from build123d import *

# Parameters (mm, degrees)
SKETCH_1_W          = 390
SKETCH_1_H          = 250
EXTRUDE_1_DEPTH     = 2
SKETCH_2_W          = 130
SKETCH_2_H          = 40
SKETCH_2_W_2        = 125
SKETCH_2_H_2        = 60
CUT_EXTRUDE_1_DEPTH = 5
CUT_EXTRUDE_2_DEPTH = 10
FILLET_1_R          = 5
SKETCH_4_R          = 1.5
SKETCH_4_R_2        = 1.75
CUT_EXTRUDE_3_DEPTH = 232.633330935
SKETCH_5_R          = 1.75
CUT_EXTRUDE_4_DEPTH = 232.633330935


with BuildPart() as part:
    # 스케치1 → 보스-돌출1 (new body)
    with BuildSketch(Plane(origin=(0, 0, 0), x_dir=(1, 0, 0), z_dir=(0, 1, 0))):
        Rectangle(SKETCH_1_W, SKETCH_1_H)
    extrude(amount=EXTRUDE_1_DEPTH)

    # 스케치2 → 컷-돌출1 (cut)
    with BuildSketch(Plane(origin=(0, 2, 0), x_dir=(1, 0, 0), z_dir=(0, 1, 0))):
        with Locations((-85, 105)):
            Rectangle(SKETCH_2_W, SKETCH_2_H)
        with Locations((-85, -105)):
            Rectangle(SKETCH_2_W, SKETCH_2_H)
        with Locations((132.5, 95)):
            Rectangle(SKETCH_2_W_2, SKETCH_2_H_2)
        with Locations((132.5, -95)):
            Rectangle(SKETCH_2_W_2, SKETCH_2_H_2)
    extrude(amount=-CUT_EXTRUDE_1_DEPTH, mode=Mode.SUBTRACT)

    # 스케치3 → 컷-돌출2 (cut)
    with BuildSketch(Plane(origin=(0, 2, 0), x_dir=(1, 0, 0), z_dir=(0, 1, 0))):
        Polygon((-5, 125), (70, 65), (70, 125), align=None)
        Polygon((70, -65), (-5, -125), (70, -125), align=None)
    extrude(amount=-CUT_EXTRUDE_2_DEPTH, mode=Mode.SUBTRACT)

    # 필렛1
    fillet_1_edges = [part.edges().sort_by_distance(p)[0] for p in [
        (-5, 1, -125),
        (-5, 1, 125),
        (-150, 1, 125),
        (-20, 1, 125),
        (195, 1, -65),
        (195, 1, 65),
        (-150, 1, -125),
        (-20, 1, -125),
        (-195, 1, 125),
        (-195, 1, -125),
    ]]
    fillet(fillet_1_edges, radius=FILLET_1_R)

    # 스케치4 → 컷-돌출3 (cut, through all)
    with BuildSketch(Plane(origin=(0, 2, 0), x_dir=(1, 0, 0), z_dir=(0, 1, 0))):
        with Locations(Location((-100, 77, 0), (0, 0, 270))):
            Circle(SKETCH_4_R)
        with Locations(Location((-70, 77, 0), (0, 0, 270))):
            Circle(SKETCH_4_R)
        with Locations(Location((-70, 53, 0), (0, 0, 270))):
            Circle(SKETCH_4_R)
        with Locations(Location((-100, 53, 0), (0, 0, 270))):
            Circle(SKETCH_4_R)
        with Locations(Location((-100, -53, 0), (0, 0, 90))):
            Circle(SKETCH_4_R)
        with Locations(Location((-70, -53, 0), (0, 0, 90))):
            Circle(SKETCH_4_R)
        with Locations(Location((-70, -77, 0), (0, 0, 90))):
            Circle(SKETCH_4_R)
        with Locations(Location((-100, -77, 0), (0, 0, 90))):
            Circle(SKETCH_4_R)
        with Locations(Location((100, 60, 0), (0, 0, 270))):
            Circle(SKETCH_4_R_2)
        with Locations(Location((110, 60, 0), (0, 0, 270))):
            Circle(SKETCH_4_R_2)
        with Locations(Location((100, 10, 0), (0, 0, 270))):
            Circle(SKETCH_4_R_2)
        with Locations(Location((110, 10, 0), (0, 0, 270))):
            Circle(SKETCH_4_R_2)
        with Locations(Location((100, -10, 0), (0, 0, 270))):
            Circle(SKETCH_4_R_2)
        with Locations(Location((110, -10, 0), (0, 0, 270))):
            Circle(SKETCH_4_R_2)
        with Locations(Location((100, -60, 0), (0, 0, 270))):
            Circle(SKETCH_4_R_2)
        with Locations(Location((110, -60, 0), (0, 0, 270))):
            Circle(SKETCH_4_R_2)
    extrude(amount=-CUT_EXTRUDE_3_DEPTH, mode=Mode.SUBTRACT)

    # 스케치5 → 컷-돌출4 (cut, through all)
    with BuildSketch(Plane(origin=(0, 2, 0), x_dir=(1, 0, 0), z_dir=(0, 1, 0))):
        with Locations(Location((-13, -8.5, 0), (0, 0, 270))):
            Circle(SKETCH_5_R)
        with Locations(Location((35, -8.5, 0), (0, 0, 270))):
            Circle(SKETCH_5_R)
        with Locations(Location((-13, -26.5, 0), (0, 0, 270))):
            Circle(SKETCH_5_R)
        with Locations(Location((35, -26.5, 0), (0, 0, 270))):
            Circle(SKETCH_5_R)
    extrude(amount=-CUT_EXTRUDE_4_DEPTH, mode=Mode.SUBTRACT)


solid = part.part
Input: part model. Units: mm. Frame: model coordinates. Round coordinates to 2 decimals unless told otherwise and drop trailing zeros. Order: outer loops, then holes, each group sorted by start corner. A loop starts at its lowest first (then second) coordinate and runs counter-clockwise, first axis right, second up. Notation, with made-up numbers: (-16.75, 50) - (41.25, 50) arc R19 ccw to (41.25, 72) - close; hole circle Ø11 at (61, 40.5). An arc over 180 degrees is marked (long way). Answer as a JSON object with one key per item and string values. Group by question number.
(1) Cut plane B-B (x = -50). Return loops of the section in (y, z), then the cut area to 3 significant figures.
(2) Material intervals for probe 1 along X at (y, z) = (0.6, -53); probe 2 along X at (y, z) = (0.8, -60); probe 3 along Z at (x, y) = (109, 0.2), sorted ascending. Write a range as from..to.
(3) Cut plane A-A (y = 0.95). Count the separate pieces of the cut face and the enclosed holes in it, then the cut area to 3 significant figures.
(4) Pin query (flat end, axial travel): P1, Ø1.8, axis at x = -100, z = 53, coming from the -Y side; P2, Ø3.5, axis at x = -70, z = -53, coming from the +Y side; P3, Ø1, axis at x = -83, y = 1.5, coming from the -Z side; P4, Ø0.6, axis at y = 1, z = -100.5, coming from the +X side. Return the tip coordinate at first contact, or that it passes through.
Here are the results:
{
 "1": {"outline": "(0, -85) - (2, -85) - (2, 85) - (0, 85) - close", "area": "340 mm^2"},
 "2": {"probe 1": "x = -195..-101.5, -98.5..-71.5, -68.5..195", "probe 2": "x = -195..98.25, 101.75..108.25, 111.75..195", "probe 3": "z = -65..-61.44, -58.56..-11.44, -8.56..8.56, 11.44..58.56, 61.44..65"},
 "3": {"separate pieces": "1", "enclosed holes": "20", "area": "67,400 mm^2"},
 "4": {"P1": "passes through", "P2": "stops at y = 2", "P3": "stops at z = -85", "P4": "stops at x = 26"}
}
